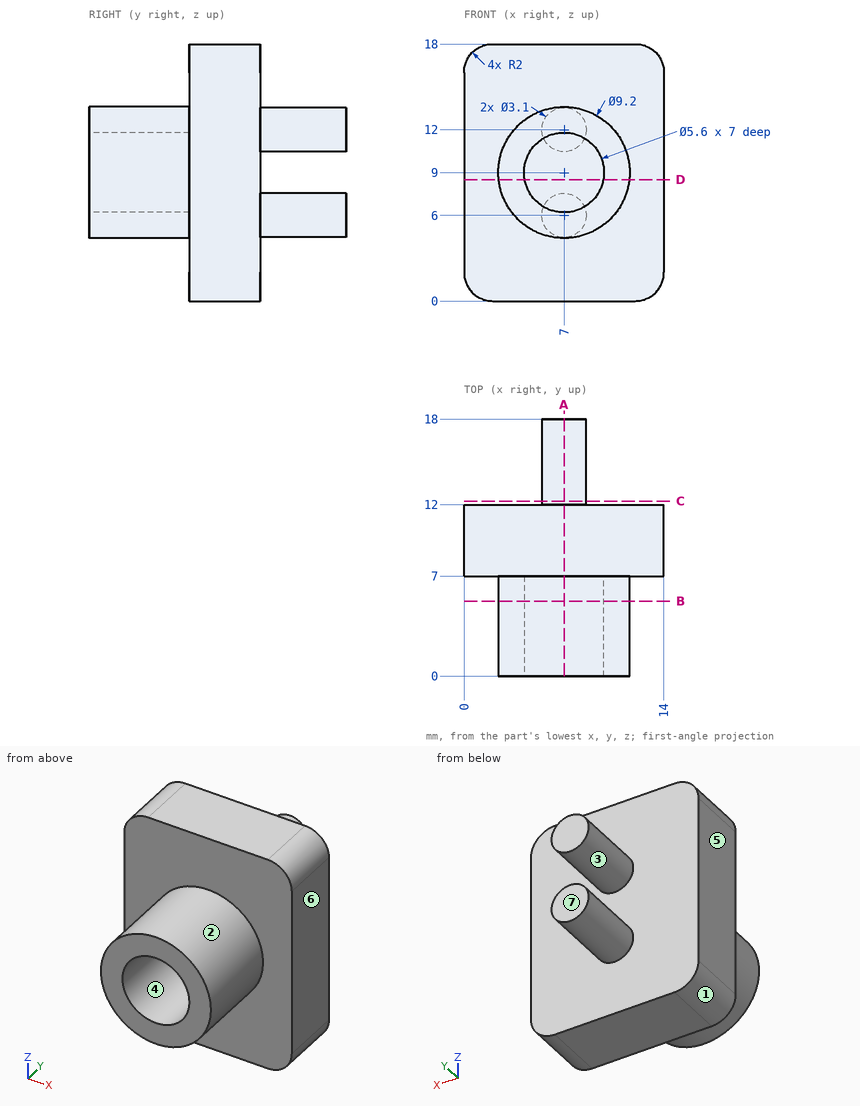
Study the drawing (mm; zero at the part's minimum x, y, z) and answer. A direction names the side the tool comes from. Round coordinates to 2 decimals unless told otherwise and drop trailing zeros. Loops run counter-clockwise (first coordinate to the right, second up) from the corner with the lowest first, then second, coordinate; pieces in that order, holes last. Notation, with made-up numbers: (61, -2.75) - (120, -2.75) arc R19 cw to (120, 11.25) - close; hole circle Ø11 at (36, -40). An arc over 180 degrees is marked (long way). Use one line per item in the form item = value. Start each with the question number.
1. The part is cut by section B-B on y = 5.25. Determine the outline of the cut face in (x, z), then the cut area to 3 significant figures.
2. For a pull along X with two mould halves and no side action, classify the marked faces 4, 5, 6 and 7 as pulls with the +X half, pulls with the -X half, needs draft (parallel to the pull), parting line crosses it, or undercut.
3. The part is cut by section D-D on z = 8.5. Determine the outline of the cut face in (x, y) (3 decimals), then the cut area to 3 significant figures.
4. Consider line 1 (X direction, y = 4.25, z = 9); line 2 (Z direction, x = 7, y = 4); line 3 (Y direction, x = 6, z = 11.5). Determine where each line is inside the solid, lowest interval first. Write a range as [from, to].
5. Given pin 1 Ø1.7 at (x, z) = (6, 8.5) entering from -Y; pin 2 Ø1 at (x, y) = (6.5, 14) entering from +Z; pin 3 Ø2 at (x, z) = (3.5, 12.5) entering from +Y, each flat-ended and moving along its own axis, determine where each tip first touches the part or whether it passes through.
6. The part is cut by section A-A on x = 7. Determine the outline of the cut face in (y, z).
7. A tool of negligible diameter and unlimited length cuts with its end or side. For the marked faces 1, 2 and 3, from which of +Z, -Z, +X, -X, +Y, -Y can it reach the whole face along a straight path? Write none if from no direction.
8. The part is cut by section C-C on y = 12.25. Determine the outline of the cut face in (x, z), then the cut area to 3 significant figures.
Geometry check:
q1.outline = circle Ø9.2 at (7, 9); hole circle Ø5.6 at (7, 9)
q1.area = 41.8 mm^2
q2.face_4 = undercut
q2.face_5 = pulls with the -X half
q2.face_6 = pulls with the +X half
q2.face_7 = needs draft
q3.outline = (0, 7) - (2.427, 7) - (2.427, 0) - (4.245, 0) - (4.245, 7) - (9.755, 7) - (9.755, 0) - (11.573, 0) - (11.573, 7) - (14, 7) - (14, 12) - (0, 12) - close
q3.area = 95.4 mm^2
q4.line_1 = [2.4, 4.2], [9.8, 11.6]
q4.line_2 = [4.4, 6.2], [11.8, 13.6]
q4.line_3 = [7, 18]
q5.pin_1 = 7
q5.pin_2 = 13.55
q5.pin_3 = 12
q6.outline = (0, 4.4) - (7, 4.4) - (7, 0) - (12, 0) - (12, 4.45) - (18, 4.45) - (18, 7.55) - (12, 7.55) - (12, 10.45) - (18, 10.45) - (18, 13.55) - (12, 13.55) - (12, 18) - (7, 18) - (7, 13.6) - (0, 13.6) - (0, 11.8) - (7, 11.8) - (7, 6.2) - (0, 6.2) - close
q7.face_1 = -Z, -X, +Y, -Y
q7.face_2 = -Y
q7.face_3 = +Y
q8.outline = circle Ø3.1 at (7, 6); circle Ø3.1 at (7, 12)
q8.area = 15.1 mm^2
